Check sheet for the modelled part. Datum: model origin and axes. Units: mm. Face numbers are marked on the shaded views. A direction names the side the tool comes from. Coordinates: 2 decimals unless noted, no trailing zeros. Order: outer loops, then holes, each group sorted by start corner. A loop starts at its lowest first (then second) coordinate and runs counter-clockwise, first axis right, second up.
1. Thickness scan on line 1 (Z direction, x = 7, y = 0.5); line 2 (Z direction, x = -2.5, y = -14.75); line 3 (Y direction, x = -1.25, z = 2.5). Record the ranges inside material, lowest first.
2. Cross-section at B-B (x = 0). Enter the section's corners in (y, z).
3. Cross-section at D-D (y = -0.5). Enter the section's corners in (x, z).
4. Set-up check for the marked faces 1, 2, 3 and 4: record each of +Z, -Z, +X, -X, +Y, -Y from which the full face is reachable in a straight line by a thin tool's end or side.
5. Gauge pin test, flat ends, axial feed: pin 1 Ø2.5 at (x, y) = (0.5, -13) entering from -Z; pin 2 Ø3 at (x, z) = (1.5, 14) entering from +Y; pin 3 Ø0.6 at (x, y) = (-1, -9) entering from +Z; pin 4 Ø3 at (x, y) = (-1.5, -12.5) entering from -Z. Record the tip position at first contact, or that the pin passes through.
6. Cross-section at C-C (z = 3.75). Enter the section's corners in (x, y), then the cut area to 3 significant figures.
7. Cross-section at A-A (y = -14.5). Enter the section's corners in (x, z).
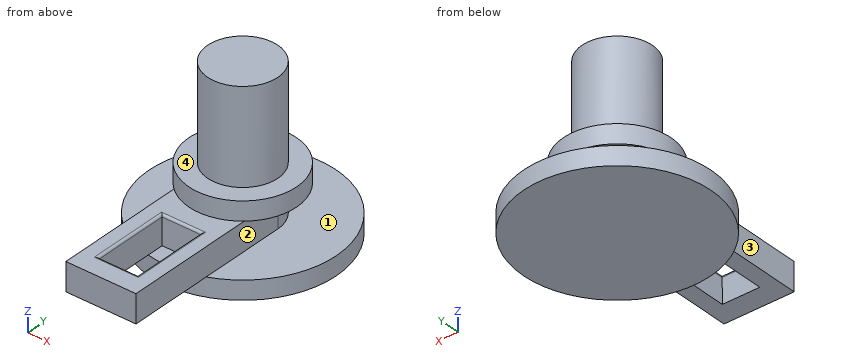
Autodesk Inventor part; units mm, degrees
ref_plane "Work Plane2" through (0, 0, 7) normal (0, 0, 1) x (1, 0, 0)
ref_plane "YZ Plane" through (0, 0, 0) normal (1, 0, 0) x (0, 1, 0)
ref_plane "XZ Plane" through (0, 0, 0) normal (0, 1, 0) x (-1, 0, 0)
sketch "Sketch1" plane through (0, 0, 0) normal (0, 0, 1) x (1, 0, 0)
  circle A0 centre (0, 0) radius 10
  dimension "d0" = 20
extrude "Extrusion1" add sketch "Sketch1" along normal blind 2
sketch "Sketch2" plane through (0, 0, 2) normal (0, 0, 1) x (1, 0, 0)
  circle A0 centre (0, 0) radius 3.75
  dimension "d3" = 7.5
extrude "Extrusion2" add sketch "Sketch2" along normal blind 15
ref_plane "Work Plane2" through (0, 0, 7) normal (0, 0, 1) x (1, 0, 0)
sketch "Sketch7" plane through (0, 0, 7) normal (0, 0, 1) x (1, 0, 0)
  circle A0 centre (0, 0) radius 3.75
  circle A1 centre (0, 0) radius 5.75
  dimension "d27" = 2
extrude "Extrusion7" add sketch "Sketch7" against normal blind 2
sketch "Sketch8" plane through (0, 0, 5) normal (0, 0, -1) x (-1, 0, 0)
  circle A0 centre (0, 0) radius 5.75
  circle A1 centre (0, 0) radius 3.75
  circle A2 centre (0, 0) radius 5.75 construction
  line L0 (5.75, 0) -> (-5.75, 0) construction
  line L1 (-3.75, 0) -> (3.75, 0)
  line L2 (3.75, 0) -> (3.75, -18.3333)
  line L3 (3.75, -18.3333) -> (-3.75, -18.3333)
  line L4 (-3.75, -18.3333) -> (-3.75, 0)
  dimension "d31" = 18.3333
extrude "Extrusion8" add sketch "Sketch8" along normal blind 3 contours L4 A1 L2 A0 | A0 L2 L3 L4 picked at (2.8343, -4.1874)
sketch "Sketch9" plane through (0, 0, 2) normal (0, 0, -1) x (-1, 0, 0)
  arc A0 (-3.75, -4.3589) -> (3.75, -4.3589) centre (0, 0) ccw
  line L0 (3.75, -18.3333) -> (3.75, -4.3589)
  line L1 (-3.75, -18.3333) -> (3.75, -18.3333)
  line L2 (-3.75, -4.3589) -> (-3.75, -18.3333)
  line L3 (-2, -8) -> (2, -8)
  line L4 (2, -8) -> (2, -16)
  line L5 (2, -16) -> (-2, -16)
  line L6 (-2, -16) -> (-2, -8)
  dimension "d34" = 2
  dimension "d35" = 4
  dimension "d36" = 8
  dimension "d37" = 8
extrude "Extrusion9" cut sketch "Sketch9" against normal up to surface (3 mm away) draft 2 contours L3 L4 L5 L6
fillet "Fillet2" radius 0.25 4 edges at (0, -16.1048, 5) (2.1048, -12, 5) (-2.1048, -12, 5) (0, -7.8952, 5)
equation "\"d1\" = IG_gearThickness"
equation "\"d3\" = IG_shaftDiameter"
equation "\"d4\" = IG_shaftLength"
equation "\"Wheel_Related_W_\" = 0"
equation "\"W_innerDepth\" = 4"
equation "\"W_wallThickness\" = 2"
equation "\"W_holesClearance\" = 0.3"
equation "\"W_outerGearHoleDiameter\" = 5.3"
equation "\"W_innerGearHoleDiameter\" = 10.1"
equation "\"TempSpotReserved7\" = 0"
equation "\"TempSpotReserved8\" = 0"
equation "\"TempSpotReserved9\" = 0"
equation "\"TempSpotReserved10\" = 0"
equation "\"TempSpotReserved11\" = 0"
equation "\"TempSpotReserved12\" = 0"
equation "\"TempSpotReserved13\" = 0"
equation "\"TempSpotReserved14\" = 0"
equation "\"TempSpotReserved15\" = 0"
equation "\"TempSpotReserved16\" = 0"
equation "\"TempSpotReserved17\" = 0"
equation "\"TempSpotReserved18\" = 0"
equation "\"TempSpotReserved19\" = 0"
equation "\"TempSpotReserved20\" = 0"
equation "\"Inner_Gear_Related_IG_\" = 0"
equation "\"IG_shaftDiameter\" = 7.5"
equation "\"IG_shaftLength\" = 15"
equation "\"IG_gearThickness\" = 2"
equation "\"TempSpotReserved25\" = 0"
equation "\"TempSpotReserved26\" = 0"
equation "\"TempSpotReserved27\" = 0"
equation "\"TempSpotReserved28\" = 0"
equation "\"TempSpotReserved29\" = 0"
equation "\"TempSpotReserved30\" = 0"
equation "\"TempSpotReserved31\" = 0"
equation "\"TempSpotReserved32\" = 0"
equation "\"TempSpotReserved33\" = 0"
equation "\"TempSpotReserved34\" = 0"
equation "\"TempSpotReserved35\" = 0"
equation "\"TempSpotReserved36\" = 0"
equation "\"TempSpotReserved37\" = 0"
equation "\"TempSpotReserved38\" = 0"
equation "\"TempSpotReserved39\" = 0"
equation "\"TempSpotReserved40\" = 0"
equation "\"Outer_Gear_Related_OG_\" = 0"
equation "\"OG_distanceFromCenter\" = 23.33333"
equation "\"OG_shaftDiameter\" = 5"
equation "\"OG_gearDiameter\" = 26.66667"
equation "\"OG_shaftLength\" = 7"
equation "\"OG_gearThickness\" = 2"
equation "\"TempSpotReserved47\" = 0"
equation "\"TempSpotReserved48\" = 0"
equation "\"TempSpotReserved49\" = 0"
equation "\"TempSpotReserved50\" = 0"
equation "\"TempSpotReserved51\" = 0"
equation "\"TempSpotReserved52\" = 0"
equation "\"TempSpotReserved53\" = 0"
equation "\"TempSpotReserved54\" = 0"
equation "\"TempSpotReserved55\" = 0"
equation "\"TempSpotReserved56\" = 0"
equation "\"TempSpotReserved57\" = 0"
equation "\"TempSpotReserved58\" = 0"
equation "\"TempSpotReserved59\" = 0"
equation "\"TempSpotReserved60\" = 0"
equation "\"Leg_Extensions_Related_LE_\" = 0"
equation "\"LE_baseDiameter\" = 5"
equation "\"LE_maxLength\" = 24.6522"
equation "\"LE_thickness\" = 2.5"
equation "\"IG_ratioToOuterGear\" = 0.75"
equation "\"B_bearingThickness\" = 1"
equation "\"TempSpotReserved43\" = 0"
equation "\"TempSpotReserved45\" = 0"
equation "\"Thisisatest\" = 25.4"
equation "\"TempSpotReserved46\" = 0"
equation "\"TempSpotReserved44\" = 0"
equation "\"LE_offsetAboveOuterGear\" = 0"
equation "\"Bearing_Related_B_\" = 0"
equation "\"TempSpotReserved42\" = 0"
equation "\"OG_skirtOffset\" = 1"
equation "\"OG_skirtThickness\" = 1"
equation "\"IG_skirtThickness\" = 2"
equation "\"IG_extentionLength\" = 18.33333"
equation "\"IG_extentionThickness\" = 3"
equation "\"IG_slitWidth\" = 4"
equation "\"IG_slitlength\" = 8"
equation "\"IG_slitDistanceFromCenterHole\" = 8"
equation "\"IG_slitClearance\" = 0.2"
equation "\"Reserved_10\" = 0"
equation "\"Reserved_9\" = 0"
equation "\"Reserved_11\" = 0"
equation "\"Reserved_12\" = 0"
equation "\"Reserved_8\" = 0"
equation "\"Reserved_7\" = 0"
equation "\"Reserved_26\" = 0"
equation "\"Reserved_20\" = 0"
equation "\"Reserved_22\" = 0"
equation "\"Reserved_23\" = 0"
equation "\"Reserved_25\" = 0"
equation "\"Reserved_24\" = 0"
equation "\"Reserved_21\" = 0"
equation "\"Reserved_19\" = 0"
equation "\"Reserved_27\" = 0"
equation "\"Reserved_14\" = 0"
equation "\"Reserved_15\" = 0"
equation "\"Reserved_16\" = 0"
equation "\"Reserved_13\" = 0"
equation "\"Reserved_17\" = 0"
equation "\"Reserved_18\" = 0"
equation "\"Bearing_Related_BR_\" = 0"
equation "\"BR_bearingThickness\" = 1"
equation "\"Block_Related_BL_\" = 0"
equation "\"BL_width\" = 3.8"
equation "\"BL_length\" = 7.8"
equation "\"W_filletRadius\" = 0.25"
equation "\"W_extrutsionTaperAngle\" = 2deg"
equation "\"OG_protrudeDistance\" = 3"
properties part number "innerGear"
Data:
1. line 1: z = 0 to 2
1. line 2: z = 2 to 5
1. line 3: y = -18.33 to -16.02, -7.98 to 3.54
2. outline: (-18.33, 2) - (-16, 2) - (-16.1, 4.76) arc R0.25 ccw to (-16.35, 5) - (-18.33, 5) - close; (-10, 0) - (10, 0) - (10, 2) - (3.75, 2) - (3.75, 5) - (5.75, 5) - (5.75, 7) - (3.75, 7) - (3.75, 17) - (-3.75, 17) - (-3.75, 7) - (-5.75, 7) - (-5.75, 5) - (-7.65, 5) arc R0.25 ccw to (-7.9, 4.76) - (-8, 2) - (-10, 2) - close
3. outline: (-9.99, 0) - (9.99, 0) - (9.99, 2) - (3.75, 2) - (3.75, 5) - (5.73, 5) - (5.73, 7) - (3.72, 7) - (3.72, 17) - (-3.72, 17) - (-3.72, 7) - (-5.73, 7) - (-5.73, 5) - (-3.75, 5) - (-3.75, 2) - (-9.99, 2) - close
4. face 1: +Y
4. face 2: +X, +Y, -Y
4. face 3: -X, +Y, -Y
4. face 4: +Z
5. pin 1: passes through
5. pin 2: stops at y = 3.75
5. pin 3: stops at z = 2
5. pin 4: stops at z = 2
6. outline: (-3.75, -18.33) - (3.75, -18.33) - (3.75, 0) arc R3.75 ccw to (-3.75, 0) - close; hole (-2.06, -16.06) - (2.06, -16.06) - (2.06, -7.94) - (-2.06, -7.94) - close
6. area: 126 mm2
7. outline: (-3.75, 2) - (-2, 2) - (-2.1, 4.76) arc R0.25 ccw to (-2.35, 5) - (-3.75, 5) - close; (2, 2) - (3.75, 2) - (3.75, 5) - (2.35, 5) arc R0.25 ccw to (2.1, 4.76) - close
